Autodesk Inventor part; units mm, degrees
ref_plane "YZ Plane" through (0, 0, 0) normal (1, 0, 0) x (0, 1, 0)
ref_plane "XZ Plane" through (0, 0, 0) normal (0, 1, 0) x (-1, 0, 0)
ref_plane "XY Plane" through (0, 0, 0) normal (0, 0, 1) x (1, 0, 0)
sketch "草圖1" plane through (0, 0, 0) normal (0, 0, 1) x (1, 0, 0)
  line L0 (-6.7, 26.2) -> (-3, 26.2)
  line L1 (-3, 26.2) -> (-3, 17.2)
  line L2 (-3, 17.2) -> (3, 17.2)
  line L3 (3, 17.2) -> (3, 26.2)
  line L4 (3, 26.2) -> (6.7, 26.2)
  line L5 (6.7, 26.2) -> (6.7, 2)
  line L6 (-6.7, 2) -> (-6.7, 26.2)
  line L7 (-6.7, 2) -> (-4.7, 0)
  line L8 (-4.7, 0) -> (-1.5, 0)
  line L9 (6.7, 2) -> (4.7, 0)
  line L10 (4.7, 0) -> (1.5, 0)
  line L11 (-1.5, 0) -> (1.5, 0)
  point P0 (0, 0)
  point P1 (0, 17.2)
  point P2 (0, 0)
  point P3 (0, 0)
  dimension "d0" = 6
  dimension "d1" = 13.4
  dimension "d5" = 9
  dimension "d10" = 26.2
  dimension "d11" = 135
  dimension "d13" = 2
extrude "擠出1" add sketch "草圖1" along normal mid plane 7
sketch "草圖2" plane through (0, 0, 0) normal (0, 0, 1) x (1, 0, 0)
  line L0 (0, 0) -> (2.3, 0)
  line L1 (1.5, -2) -> (1.5, -10)
  line L2 (1.5, -10) -> (0, -10)
  line L3 (0, -10) -> (0, 0)
  line L4 (-4.7, 0) -> (4.7, 0) construction
  line L5 (2.3, 0) -> (2.3, -2)
  line L6 (2.3, -2) -> (1.5, -2)
  point P0 (1.5, 0)
  dimension "d20" = 4.6
  dimension "d21" = 3
  dimension "d22" = 2
  dimension "d23" = 10
revolve "迴轉1" add sketch "草圖2" angle 360 about axis through (0, -10, 0) along (0, 1, 0)
sketch "草圖3" plane through (6.7, 2, 3.5) normal (1, 0, 0) x (0, 0, -1)
  line L0 (-9.5, 11.4) -> (16.5, 11.4)
  line L1 (16.5, 11.4) -> (16.5, 5.2)
  line L2 (16.5, 5.2) -> (-9.5, 5.2)
  line L3 (-9.5, 5.2) -> (-9.5, 11.4)
  line L4 (-8.7, 8.3) -> (-4.4, 8.3) construction
  line L5 (-7.1, 6.7) -> (-6, 6.7)
  line L6 (-6, 9.9) -> (-7.1, 9.9)
  arc A0 (-7.1, 9.9) -> (-7.1, 6.7) centre (-7.1, 8.3) ccw
  arc A1 (-6, 6.7) -> (-6, 9.9) centre (-6, 8.3) ccw
  line L7 (11.4, 8.3) -> (15.7, 8.3) construction
  line L8 (13, 6.7) -> (14.1, 6.7)
  line L9 (14.1, 9.9) -> (13, 9.9)
  arc A2 (13, 9.9) -> (13, 6.7) centre (13, 8.3) ccw
  arc A3 (14.1, 6.7) -> (14.1, 9.9) centre (14.1, 8.3) ccw
  line L10 (0, -2) -> (7, -2)
  line L11 (-4.4, 8.3) -> (11.4, 8.3) construction
  point P0 (3.5, -2)
  point P1 (3.5, 5.2)
  point P2 (16.5, 8.3)
  point P3 (3.5, 8.3)
  dimension "d24" = 26
  dimension "d25" = 6.2
  dimension "d26" = 1.1
  dimension "d27" = 4.3
  dimension "d28" = 19
  dimension "d29" = 10.3
extrude "擠出2" add sketch "草圖3" against normal blind 3
properties part number "RX672-NW" material "SS41"
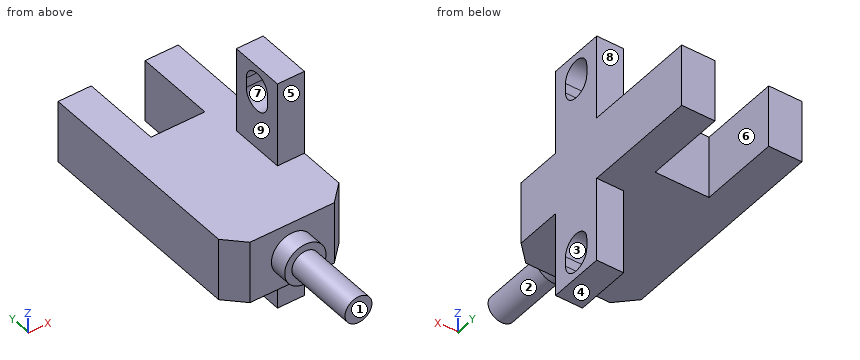
Check sheet for the modelled part. Datum: model origin and axes. Units: mm. Face numbers are marked on the shaded views. A direction names the side the tool comes from. Round coordinates to 2 decimals unless told otherwise and drop trailing zeros. Loops run counter-clockwise (first coordinate to the right, second up) from the corner with the lowest first, then second, coordinate; pieces in that order, holes last.
1. Sectioned sample at C-C on x = 5.75. Record the boundary of the cut face in (y, z), and give its area (3 significant figures).
2. Mould release check, pull along Z, two halves, no side actions. Record for the marked faces 1, 2, 3 and 4: released by +Z, released by -Z, zero draft, split by the parting line, or undercut.
3. Scan lines: probe 1 along Y at (x, z) = (4.75, -10.75); probe 2 along Z at (x, y) = (0.75, 14); probe 3 along Y at (x, z) = (-2.5, 0.25). Record each from-to range of solid material in increasing order.
4. Sectioned sample at B-B on z = -3. Record the boundary of the cut face in (x, y), and give its area (3 significant figures).
5. Gauge pin test, flat ends, axial feed: pin 1 Ø7 at (y, z) = (11.5, 7.5) entering from -X; pin 2 Ø5 at (x, z) = (0, 1.5) entering from +Y; pin 3 Ø6.5 at (x, y) = (0.5, 19.5) entering from +Z. Record the tip position at first contact, or that the pin passes through.
6. Sectioned sample at A-A on y = 18. Record the boundary of the cut face in (x, z).
7. Sectioned sample at D-D on y = 8. Record the boundary of the cut face in (x, z), and give its area (3 significant figures).
8. Set-up check for the marked faces 5, 6, 7, 8 and 9: record each of +Z, -Z, +X, -X, +Y, -Y from which the full face is reachable in a straight line by a thin tool's end or side.
Recorded:
1. outline: (1.05, -3.5) - (7.2, -3.5) - (7.2, -13) - (13.4, -13) - (13.4, -3.5) - (26.2, -3.5) - (26.2, 3.5) - (13.4, 3.5) - (13.4, 13) - (7.2, 13) - (7.2, 3.5) - (1.05, 3.5) - close; hole (8.7, -10.6) arc R1.6 ccw to (11.9, -10.6) - (11.9, -9.5) arc R1.6 ccw to (8.7, -9.5) - close; hole (8.7, 9.5) arc R1.6 ccw to (11.9, 9.5) - (11.9, 10.6) arc R1.6 ccw to (8.7, 10.6) - close
1. area: 271 mm2
2. face 1: zero draft
2. face 2: split by the parting line
2. face 3: undercut
2. face 4: released by -Z
3. probe 1: y = 7.2 to 8.71, 11.89 to 13.4
3. probe 2: z = -3.5 to 3.5
3. probe 3: y = 0 to 17.2
4. outline: (-6.7, 2) - (-4.7, 0) - (4.7, 0) - (6.7, 2) - (6.7, 26.2) - (3, 26.2) - (3, 17.2) - (-3, 17.2) - (-3, 26.2) - (-6.7, 26.2) - close
4. area: 293 mm2
5. pin 1: stops at x = 3.7
5. pin 2: stops at y = 17.2
5. pin 3: stops at z = 3.5
6. outline: (-6.7, -3.5) - (-3, -3.5) - (-3, 3.5) - (-6.7, 3.5) - close; (3, -3.5) - (6.7, -3.5) - (6.7, 3.5) - (3, 3.5) - close
7. outline: (-6.7, -3.5) - (3.7, -3.5) - (3.7, -13) - (6.7, -13) - (6.7, 13) - (3.7, 13) - (3.7, 3.5) - (-6.7, 3.5) - close
7. area: 151 mm2
8. face 5: +Z, +X, -X, -Y
8. face 6: +Z, -Z, +Y
8. face 7: +X, -X
8. face 8: +Z, +X, -X, +Y
8. face 9: +Z, -X, +Y, -Y
